Geometry: final body of the model. Coordinates: model frame, mm. A direction names the side the tool comes from. Coordinates: 2 decimals unless noted, no trailing zeros. Write each loop counter-clockwise with the first axis right and the second up, starting at its lowest first coordinate (ties: lowest second). Pieces come first, ordered by that corner, then holes. Notation, with made-up numbers: (33, 3) - (83, 3) arc R24 ccw to (83, 36) - close; hole circle Ø9 at (25, 46). An arc over 180 degrees is marked (long way). Answer as a JSON object with one key per item and string values. Group by question number.
Item 1: Line query: line 1 along Y through (x, z) = (25.5, 241); line 2 along X through (y, z) = (3, 247.5); line 3 along Y through (x, z) = (0.9, 25.4). Output: solid intervals per line, ascending. Write a range as from..to.
Item 2: Section A-A on x = 25. Return loops of the section in (y, z), and give its area (3 significant figures).
Item 3: Section C-C on z = 88.9. Return loops of the section in (x, y), and give its area (3 significant figures).
Item 4: Section B-B on y = 5.25. Return loops of the section in (x, z).
Item 5: Mould query, pull axis Y, two halves, no side actions, for faces 1 (the cylindrical face through (0.8, 15.17, 114.62)), 2 (the flat face through (25, 25.4, 138)), 3 (the flat face through (25, 0, 138)). Classes: pulls with the +Y half, pulls with the -Y half, needs draft (parallel to the pull), parting line crosses it, or undercut.
Item 6: First-contact query: pin 1 Ø3 at (y, z) = (12.7, 165.1) entering from -X. Flat tip, straight axial feed; report the tip coordinate or a pass-through.
Item 7: Set-up query: faces 4 (the flat face through (25, 23.812, 138)), 5 (the cylindrical face through (50.017, 12.809, 218.387)). Return all of +Z, -Z, +X, -X, +Y, -Y with unobstructed straight access to the full face (end or side cutting, diameter ignored); none if empty.
```python
from build123d import *

# Parameters (mm, degrees)
SKETCH1_W           = 50.8
SKETCH1_H           = 25.4
SKETCH1_W_2         = 47.625
SKETCH1_H_2         = 22.225
BOSS_EXTRUDE1_DEPTH = 279.4
SKETCH2_R           = 2.4892
CUT_EXTRUDE1_DEPTH  = 51.8


with BuildPart() as part:
    # Sketch1 → Boss-Extrude1 (new body)
    with BuildSketch(Plane.XY):
        with Locations((25.4, 12.7)):
            Rectangle(SKETCH1_W, SKETCH1_H)
        with Locations((25.4, 12.7)):
            Rectangle(SKETCH1_W_2, SKETCH1_H_2, mode=Mode.SUBTRACT)
    extrude(amount=BOSS_EXTRUDE1_DEPTH)

    # Sketch2 → Cut-Extrude1 (cut, through all)
    with BuildSketch(Plane(origin=(50.8, 0, 0), x_dir=(0, 0, -1), z_dir=(1, 0, 0))):
        with Locations((-266.7, 12.7)):
            Circle(SKETCH2_R)
        with Locations((-254, 12.7)):
            Circle(SKETCH2_R)
        with Locations((-241.3, 12.7)):
            Circle(SKETCH2_R)
        with Locations((-228.6, 12.7)):
            Circle(SKETCH2_R)
        with Locations((-215.9, 12.7)):
            Circle(SKETCH2_R)
        with Locations((-203.2, 12.7)):
            Circle(SKETCH2_R)
        with Locations((-190.5, 12.7)):
            Circle(SKETCH2_R)
        with Locations((-177.8, 12.7)):
            Circle(SKETCH2_R)
        with Locations((-165.1, 12.7)):
            Circle(SKETCH2_R)
        with Locations((-152.4, 12.7)):
            Circle(SKETCH2_R)
        with Locations((-139.7, 12.7)):
            Circle(SKETCH2_R)
        with Locations((-127, 12.7)):
            Circle(SKETCH2_R)
        with Locations((-114.3, 12.7)):
            Circle(SKETCH2_R)
        with Locations((-101.6, 12.7)):
            Circle(SKETCH2_R)
        with Locations((-88.9, 12.7)):
            Circle(SKETCH2_R)
        with Locations((-76.2, 12.7)):
            Circle(SKETCH2_R)
        with Locations((-63.5, 12.7)):
            Circle(SKETCH2_R)
        with Locations((-50.8, 12.7)):
            Circle(SKETCH2_R)
        with Locations((-38.1, 12.7)):
            Circle(SKETCH2_R)
        with Locations((-25.4, 12.7)):
            Circle(SKETCH2_R)
        with Locations((-12.7, 12.7)):
            Circle(SKETCH2_R)
    extrude(amount=-CUT_EXTRUDE1_DEPTH, mode=Mode.SUBTRACT)


solid = part.part
```
Checks:
{
 "1": {"line 1": "0..1.59, 23.81..25.4", "line 2": "0..1.59, 49.21..50.8", "line 3": "0..10.21, 15.19..25.4"},
 "2": {"outline": "(0, 0) - (1.59, 0) - (1.59, 279.4) - (0, 279.4) - close; (23.81, 0) - (25.4, 0) - (25.4, 279.4) - (23.81, 279.4) - close", "area": "887 mm^2"},
 "3": {"outline": "(0, 0) - (50.8, 0) - (50.8, 10.21) - (49.21, 10.21) - (49.21, 1.59) - (1.59, 1.59) - (1.59, 10.21) - (0, 10.21) - close; (0, 15.19) - (1.59, 15.19) - (1.59, 23.81) - (49.21, 23.81) - (49.21, 15.19) - (50.8, 15.19) - (50.8, 25.4) - (0, 25.4) - close", "area": "216 mm^2"},
 "4": {"outline": "(0, 0) - (1.59, 0) - (1.59, 279.4) - (0, 279.4) - close; (49.21, 0) - (50.8, 0) - (50.8, 279.4) - (49.21, 279.4) - close"},
 "5": {"face 1": "undercut", "face 2": "pulls with the +Y half", "face 3": "pulls with the -Y half"},
 "6": {"pin 1": "through"},
 "7": {"face 4": "+Z, -Z", "face 5": "+X, -X"}
}
